Geometry check sheet. Reference: the model listing, model coordinates, mm. Face numbers are marked on the shaded views. A direction names the side the tool comes from. Give positions to 0.01 mm unless a question says otherwise; leave off trailing zeros. Write each loop counter-clockwise with the first axis right and the second up, starting at its lowest first coordinate (ties: lowest second). Pieces come first, ordered by that corner, then holes. Notation, with made-up numbers: M -25.75,-32 L -21.75,-32 A18 ccw -21.75,-6 Z; hole C -35.5,27.25 d1. An arc over 180 degrees is marked long. One line per item, written item: value. Start each with the question number.
1. Release check for a two-part mould opening along Y. For the marked faces 1, 2 and 3 record: pulls with the +Y half, pulls with the -Y half, needs draft (parallel to the pull), parting line crosses it, or undercut.
2. Tool access check on the marked faces 4, 5 and 6. Record the directions out of +Z, -Z, +X, -X, +Y, -Y that give a thin tool (end or side, any length) a straight path to the whole face; none if there is none.
3. Cross-section at D-D on z = 0. Record the cut outline in (x, y) (3 decimals).
4. Cross-section at A-A on y = -76.5. Record the cut outline in (x, z).
5. Cross-section at B-B on x = 93.5. Record the cut outline in (y, z).
6. Gauge pin test, flat ends, axial feed: pin 1 (10 mm diameter, centred on x = -57, z = -19.5, fed in from -Y); pin 2 (6 mm diameter, centred on x = 59, z = -17, fed in from +Y); pin 3 (4 mm diameter, centred on x = 79, z = -7.5, fed in from +Y). Record the tip position at first contact, or that the pin passes through.
7. Scan lines: line 1 (X direction, y = -12, z = 0) (3 decimals); line 2 (X direction, y = -70, z = 0); line 3 (Y direction, x = -0.5, z = -6). Record each from-to range of solid material in increasing order.
8. Cross-section at C-C on y = -25.5. Record the cut outline in (x, z) (3 decimals), then the cut area to 3 significant figures.
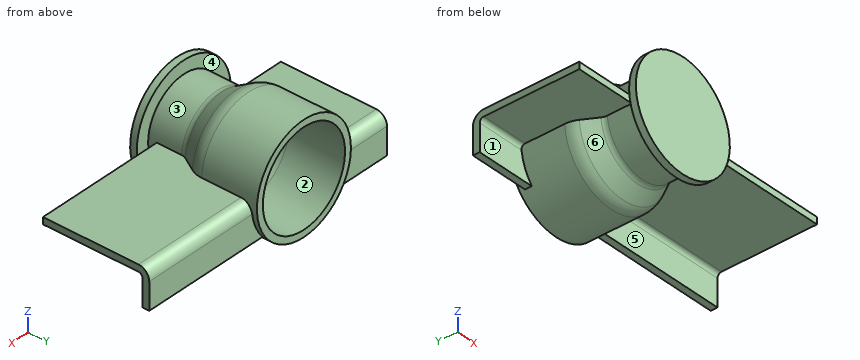
from build123d import *

# Parameters (mm, degrees)
EXTRUDE_1_REACH   = 195.29
SKETCH_3_R        = 39.925
EXTRUDE_1_2_DEPTH = 5
EXTRUDE_3_REACH   = 228.308


with BuildPart() as part:
    # strainer → 旋轉-薄件1 (revolve)
    with BuildSketch(Plane.XY, mode=Mode.PRIVATE) as revolve_1_sk:
        with BuildLine():
            Line((-34.925, 0), (-34.925, -41.047045184))
            ThreePointArc((-34.925, -41.047045184), (-34.492257994, -44.334047057), (-33.223522628, -47.397045184))
            Line((-33.223522628, -47.397045184), (-27.101477372, -58.000738614))
            ThreePointArc((-27.101477372, -58.000738614), (-25.832742006, -61.063736741), (-25.4, -64.350738614))
            Line((-25.4, -64.350738614), (-25.4, -88.9))
            Line((-25.4, -88.9), (-30.4, -88.9))
            Line((-30.4, -88.9), (-30.4, -64.350738614))
            ThreePointArc((-30.4, -64.350738614), (-30.662371138, -62.357831967), (-31.431604391, -60.500738614))
            Line((-31.431604391, -60.500738614), (-37.553649647, -49.897045184))
            ThreePointArc((-37.553649647, -49.897045184), (-39.321887125, -45.628142282), (-39.925, -41.047045184))
            Line((-39.925, -41.047045184), (-39.925, 0))
            Line((-39.925, 0), (-34.925, 0))
        make_face()
    revolve(revolve_1_sk.sketch.rotate(Axis((0, 0, 0), (0, 1, 0)), 270), axis=Axis((0, 0, 0), (0, 1, 0)))

    # bracket → Extrude 1 (add, up to next)
    with BuildSketch(Plane(origin=(127, 0, 0), x_dir=(0, 0, -1), z_dir=(1, 0, 0)), mode=Mode.PRIVATE) as extrude_1_sk1:
        with BuildLine():
            Line((25.4, -3.85), (5.5, -3.85))
            ThreePointArc((5.5, -3.85), (-0.156854249, -6.193145751), (-2.5, -11.85))
            Line((-2.5, -11.85), (-2.5, -82.55))
            Line((-2.5, -82.55), (2.5, -82.55))
            Line((2.5, -82.55), (2.5, -11.85))
            ThreePointArc((2.5, -11.85), (3.378679656, -9.728679656), (5.5, -8.85))
            Line((5.5, -8.85), (25.4, -8.85))
            Line((25.4, -8.85), (25.4, -3.85))
        make_face()
    extrude_1_tool1 = extrude(extrude_1_sk1.sketch, amount=-EXTRUDE_1_REACH, mode=Mode.PRIVATE) - part.part
    add(extrude_1_tool1.solids().sort_by_distance((127, -4.684991, -15.45))[0])

    # 草圖3 → Extrude 1 2 (add)
    with BuildSketch(Plane.XZ.offset(88.9)):
        with Locations(Location((0, 0, 0), (0, 0, 270))):
            Circle(SKETCH_3_R)
    extrude(amount=EXTRUDE_1_2_DEPTH)

    # 草圖4 → 填料-伸長3 (add, up to next)
    with BuildSketch(Plane(origin=(-75, 0, 0), x_dir=(0, 0, -1), z_dir=(1, 0, 0)), mode=Mode.PRIVATE) as extrude_3_sk1:
        with BuildLine():
            Line((5.5, -8.85), (25.4, -8.85))
            Line((25.4, -8.85), (25.4, -3.85))
            Line((25.4, -3.85), (5.5, -3.85))
            ThreePointArc((5.5, -3.85), (-0.156854249, -6.193145751), (-2.5, -11.85))
            Line((-2.5, -11.85), (-2.5, -82.55))
            Line((-2.5, -82.55), (2.5, -82.55))
            Line((2.5, -82.55), (2.5, -11.85))
            ThreePointArc((2.5, -11.85), (3.378679656, -9.728679656), (5.5, -8.85))
        make_face()
    extrude_3_tool1 = extrude(extrude_3_sk1.sketch, amount=EXTRUDE_3_REACH, mode=Mode.PRIVATE) - part.part
    add(extrude_3_tool1.solids().sort_by_distance((-75, -9.138252, -2.788252))[0])


solid = part.part
Report:
1. face 1: pulls with the -Y half
1. face 2: needs draft
1. face 3: undercut
2. face 4: none
2. face 5: -Z, +X, -Y
2. face 6: -Z
3. outline: M -75,-82.55 L -30.4,-82.55 L -30.4,-88.9 L -39.925,-88.9 L -39.925,-93.9 L 39.925,-93.9 L 39.925,-88.9 L 30.4,-88.9 L 30.4,-82.55 L 127,-82.55 L 127,-6.041 L 39.925,-6.041 L 39.925,0 L 34.925,0 L 34.925,-41.047 A12.7 cw 33.224,-47.397 L 27.101,-58.001 A12.7 ccw 25.4,-64.351 L 25.4,-88.9 L -25.4,-88.9 L -25.4,-64.351 A12.7 ccw -27.101,-58.001 L -33.224,-47.397 A12.7 cw -34.925,-41.047 L -34.925,0 L -39.925,0 L -39.925,-6.041 L -75,-6.041 Z
4. outline: M -75,-2.5 L -30.3,-2.5 A30.4 ccw 30.3,-2.5 L 127,-2.5 L 127,2.5 L 30.3,2.5 A30.4 ccw -30.3,2.5 L -75,2.5 Z; hole C 0,0 d50.8
5. outline: M -82.55,-2.5 L -11.85,-2.5 A3 cw -8.85,-5.5 L -8.85,-25.4 L -3.85,-25.4 L -3.85,-5.5 A8 ccw -11.85,2.5 L -82.55,2.5 Z
6. pin 1: stops at y = -8.85
6. pin 2: stops at y = -3.85
6. pin 3: stops at y = -3.85
7. line 1: x = -75 to -34.925, 34.925 to 127
7. line 2: x = -75 to -25.4, 25.4 to 127
7. line 3: y = -93.9 to -88.9
8. outline: M -75,-2.5 L -39.847,-2.5 A39.925 ccw 39.847,-2.5 L 127,-2.5 L 127,2.5 L 39.847,2.5 A39.925 ccw -39.847,2.5 L -75,2.5 Z; hole C 0,0 d69.85
8. area: 1,790 mm^2
